Work out the finished part from the listing and answer in its coordinate system (mm). Face numbers are marked on the shaded views. A direction names the side the tool comes from. Round coordinates to 2 decimals unless told otherwise and drop trailing zeros. Order: outer loops, then holes, each group sorted by start corner. A loop starts at its lowest first (then second) coordinate and runs counter-clockwise, first axis right, second up. Notation, with made-up numbers: (18, 46) - (52, 46) arc R9 ccw to (52, 55) - close; hole circle Ø2 at (55, -25.75). An arc over 180 degrees is marked (long way). Put each result on its own line as item: value.
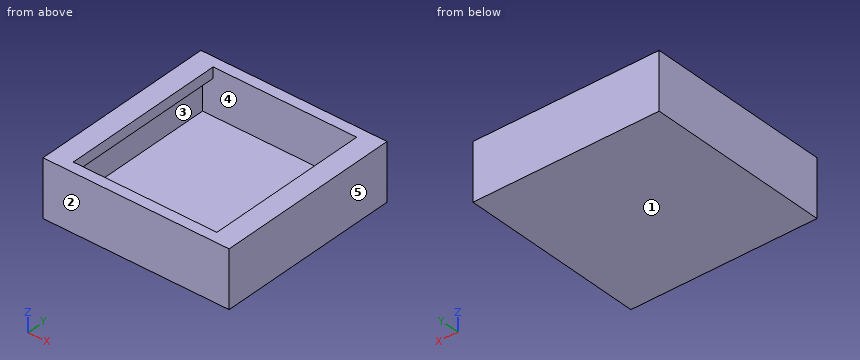
```python
from build123d import *

# Parameters (mm, degrees)
F0_W     = 52.5
F0_H     = 52.5
F1_DEPTH = 3
F2_W     = 52.5
F2_H     = 52.5
F2_W_2   = 46.5
F2_H_2   = 46.5
F3_DEPTH = 13
F4_W     = 6
F4_H     = 3
F5_DEPTH = 52.5


with BuildPart() as f1:
    # F0 (on Top) → F1 (new body)
    with BuildSketch(Plane.XY):
        Rectangle(F0_W, F0_H)
    extrude(amount=F1_DEPTH)

    # F2 (on face) → F3 (join)
    with BuildSketch(Plane.XY.offset(3)):
        Rectangle(F2_W, F2_H)
        Rectangle(F2_W_2, F2_H_2, mode=Mode.SUBTRACT)
    extrude(amount=F3_DEPTH)

    # F4 (on face) → F5 (join)
    with BuildSketch(Plane.XZ.offset(26.25)):
        with Locations((-23.25, 14.5)):
            Rectangle(F4_W, F4_H)
        with Locations((23.25, 14.5)):
            Rectangle(F4_W, F4_H)
    extrude(amount=-F5_DEPTH)


solid = f1.part
```
1) For the marked faces 4 and 5, determine the directions among +Z, -Z, +X, -X, +Y, -Y from which every point of the face is accessible in a straight line to the end or side of a thin tool.
Findings below:
face 4: none
face 5: +Z, -Z, +X, +Y, -Y
2) A cutting plane is placed at B-B on x = 22. Write down the section's boundary in (y, z).
Findings below:
outline: (-26.25, 0) - (26.25, 0) - (26.25, 16) - (-26.25, 16) - close; hole (-23.25, 3) - (23.25, 3) - (23.25, 13) - (-23.25, 13) - close
3) For a pull along Z with two mould halves and no side action, classify the marked faces 1, 2 and 3 as pulls with the +Z half, pulls with the -Z half, needs draft (parallel to the pull), parting line crosses it, or undercut.
Findings below:
face 1: pulls with the -Z half
face 2: needs draft
face 3: undercut
4) A cutting plane is placed at C-C on y = -4. Write down the section's boundary in (x, z).
Findings below:
outline: (-26.25, 0) - (26.25, 0) - (26.25, 16) - (20.25, 16) - (20.25, 13) - (23.25, 13) - (23.25, 3) - (-23.25, 3) - (-23.25, 13) - (-20.25, 13) - (-20.25, 16) - (-26.25, 16) - close
5) A cutting plane is placed at A-A on z = 9. Write down the section's boundary in (x, y).
Findings below:
outline: (-26.25, -26.25) - (26.25, -26.25) - (26.25, 26.25) - (-26.25, 26.25) - close; hole (-23.25, -23.25) - (23.25, -23.25) - (23.25, 23.25) - (-23.25, 23.25) - close
6) Straight lines are drawn through the part: L1, parallel to Y at x = -15, z = 15.25; L2, parallel to Z at x = 22, y = -19.5. For each, find the intervals that lie inside material, in ascending order. Write a range as from..to.
Findings below:
L1: y = -26.25..-23.25, 23.25..26.25
L2: z = 0..3, 13..16
